from build123d import *

# Parameters (mm, degrees)
SKETCH1_R               = 6.5
BOSS_EXTRUDE1_DEPTH     = 14
SKETCH2_R               = 2.5
BOSS_EXTRUDE2_DEPTH     = 8
CUT_EXTRUDE1_DEPTH      = 24.843238035
CUT_EXTRUDE1_DEPTH_BACK = 24.843238035
SKETCH3_R               = 4
SKETCH4_R               = 1.75
CUT_EXTRUDE2_DEPTH      = 24.843238184


with BuildPart() as part:
    # Sketch1 → Boss-Extrude1 (new body)
    with BuildSketch(Plane(origin=(0, 0, 0), x_dir=(1, 0, 0), z_dir=(0, 1, 0))):
        with Locations(Location((0, 0, 0), (0, 0, 270))):
            Circle(SKETCH1_R)
    extrude(amount=BOSS_EXTRUDE1_DEPTH)

    # Sketch2 → Boss-Extrude2 (add)
    with BuildSketch(Plane(origin=(0, 14, 0), x_dir=(1, 0, 0), z_dir=(0, 1, 0))):
        with Locations(Location((0, 0, 0), (0, 0, 270))):
            Circle(SKETCH2_R)
    extrude(amount=BOSS_EXTRUDE2_DEPTH)

    # Sketch3 → Cut-Extrude1 (cut, two sides: drawn at the far end of the back side and taken through both)
    with BuildSketch(Plane.XY.offset(-CUT_EXTRUDE1_DEPTH_BACK)):
        with Locations(Location((0, 7, 0), (0, 0, 90))):
            Circle(SKETCH3_R)
    extrude(amount=CUT_EXTRUDE1_DEPTH + CUT_EXTRUDE1_DEPTH_BACK, mode=Mode.SUBTRACT)

    # Sketch4 → Cut-Extrude2 (cut, through all)
    with BuildSketch(Plane(origin=(0, 22, 0), x_dir=(1, 0, 0), z_dir=(0, 1, 0))):
        with Locations(Location((0, 0, 0), (0, 0, 270))):
            Circle(SKETCH4_R)
    extrude(amount=-CUT_EXTRUDE2_DEPTH, mode=Mode.SUBTRACT)


solid = part.part
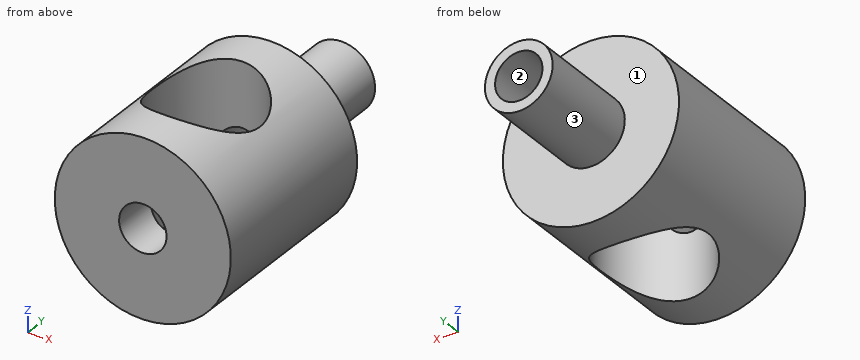
Geometry: final body of the model. Coordinates: model frame, mm. Face numbers are marked on the shaded views. Round coordinates to 2 decimals unless told otherwise and drop trailing zeros. Loops run counter-clockwise (first coordinate to the right, second up) from the corner with the lowest first, then second, coordinate; pieces in that order, holes last. Notation, with made-up numbers: (88.5, 3) -> (120.5, 3) arc R17 cw to (120.5, 8) -> close; hole circle Ø7 at (70.25, -28.75). An arc over 180 degrees is marked (long way). One line per question, with ' | ' between items. Start each with the question number.
1. Section B-B on x = 0. Output: boundary loops of the cut face in (y, z), and give its area (3 significant figures).
2. Section D-D on y = 18.5. Output: boundary loops of the cut face in (x, z).
3. Mould query, pull axis Z, two halves, no side actions, for the marked faces 1, 2 and 3. Classes: pulls with the +Z half, pulls with the -Z half, needs draft (parallel to the pull), parting line crosses it, or undercut.
4. Contact query for flat-ended pins moving along their axis: pin 1 (3 mm diameter, centred on x = -3, y = 15, fed in from +Z); pin 2 (1.5 mm diameter, centred on x = 0, z = -5, fed in from +Y); pin 3 (1 mm diameter, centred on x = 5, y = 8, fed in from -Z). Output: stop coordinate, or through.
5. Line query: line 1 along X through (y, z) = (1.25, 0); line 2 along Y through (x, z) = (-3.5, -2.75); line 3 along Y through (x, z) = (-1.5, -6). Output: solid intervals per line, ascending. Write a range as [from, to].
6. Section C-C on x = 3.5. Output: boundary loops of the cut face in (y, z).
7. Section A-A on z = 0. Output: boundary loops of the cut face in (x, y).
Returned:
1) outline: (0, -6.5) -> (3, -6.5) -> (3, -1.75) -> (0, -1.75) -> close; (0, 1.75) -> (3, 1.75) -> (3, 6.5) -> (0, 6.5) -> close; (11, -6.5) -> (14, -6.5) -> (14, -2.5) -> (22, -2.5) -> (22, -1.75) -> (11, -1.75) -> close; (11, 1.75) -> (22, 1.75) -> (22, 2.5) -> (14, 2.5) -> (14, 6.5) -> (11, 6.5) -> close | area: 69.0 mm2
2) outline: circle Ø5 at (0, 0); hole circle Ø3.5 at (0, 0)
3) face 1: needs draft | face 2: undercut | face 3: parting line crosses it
4) pin 1: stops at z = 6.22 | pin 2: stops at y = 14 | pin 3: stops at z = -4.69
5) line 1: x = [-6.5, -1.75], [1.75, 6.5] | line 2: y = [0, 5.06], [8.94, 14] | line 3: y = [0, 3.29], [10.71, 14]
6) outline: (0, -5.48) -> (5.06, -5.48) -> (5.06, 5.48) -> (0, 5.48) -> close; (8.94, -5.48) -> (14, -5.48) -> (14, 5.48) -> (8.94, 5.48) -> close
7) outline: (-6.5, 0) -> (-1.75, 0) -> (-1.75, 3.4) arc R4 cw to (-1.75, 10.6) -> (-1.75, 22) -> (-2.5, 22) -> (-2.5, 14) -> (-6.5, 14) -> close; (1.75, 0) -> (6.5, 0) -> (6.5, 14) -> (2.5, 14) -> (2.5, 22) -> (1.75, 22) -> (1.75, 10.6) arc R4 cw to (1.75, 3.4) -> close
